```python
from build123d import *

# Parameters (mm, degrees)
P01_CONTACTTOPLEG_START = 37
SK_P01_CONTACTTOPLEG_W  = 25
SK_P01_CONTACTTOPLEG_H  = 24
P01_CONTACTTOPLEG_DEPTH = 3
SK_P02_CONTACTFACE_W    = 3
SK_P02_CONTACTFACE_H    = 24
P02_CONTACTFACE_DEPTH   = 37


with BuildPart() as part:
    # SK_P01_Contacttopleg → P01_Contacttopleg (new body)
    with BuildSketch(Plane(origin=(0, 0, 0), x_dir=(1, 0, 0), z_dir=(0, 1, 0)).offset(P01_CONTACTTOPLEG_START)):
        Rectangle(SK_P01_CONTACTTOPLEG_W, SK_P01_CONTACTTOPLEG_H)
    extrude(amount=P01_CONTACTTOPLEG_DEPTH)

    # SK_P02_Contactface → P02_Contactface (add)
    with BuildSketch(Plane(origin=(0, 0, 0), x_dir=(1, 0, 0), z_dir=(0, 1, 0))):
        with Locations((11, 0)):
            Rectangle(SK_P02_CONTACTFACE_W, SK_P02_CONTACTFACE_H)
    extrude(amount=P02_CONTACTFACE_DEPTH)


solid = part.part
```
Input: part model. Units: mm. Frame: model coordinates. A direction names the side the tool comes from. Round coordinates to 2 decimals unless told otherwise and drop trailing zeros. Order: outer loops, then holes, each group sorted by start corner. A loop starts at its lowest first (then second) coordinate and runs counter-clockwise, first axis right, second up. Notation, with made-up numbers: (-36, 70) - (-10, 70) arc R10 ccw to (-10, 88) - close; hole circle Ø7 at (6.25, 50). An arc over 180 degrees is marked (long way). Answer in a Markdown table with one row per item.
Item 1: Section query B-B (y = 16.5). Return the cut outline in (x, z), then the cut area to 3 significant figures.
Model answer:
| item | result |
|---|---|
| outline | (9.5, -12) - (12.5, -12) - (12.5, 12) - (9.5, 12) - close |
| area | 72.0 mm² |
Item 2: Line query: line 1 (Y direction, x = -2.5, z = 2.75); line 2 (X direction, y = 16, z = 7). Output: solid intervals per line, ascending.
Model answer:
| item | result |
|---|---|
| line 1 | y = 37 to 40 |
| line 2 | x = 9.5 to 12.5 |
Item 3: Pin query (flat end, axial travel): pin 1 (3 mm diameter, centred on x = -9.5, z = 2, fed in from -Y); pin 2 (10 mm diameter, centred on y = 23.5, z = -1, fed in from -X). Return the tip coordinate at first contact, or that it passes through.
Model answer:
| item | result |
|---|---|
| pin 1 | stops at y = 37 |
| pin 2 | stops at x = 9.5 |
Item 4: Section query A-A (z = -8.5). Return the cut outline in (x, y).
Model answer:
| item | result |
|---|---|
| outline | (-12.5, 37) - (9.5, 37) - (9.5, 0) - (12.5, 0) - (12.5, 40) - (-12.5, 40) - close |
Item 5: Section query C-C (x = 1.5). Return the cut outline in (y, z).
Model answer:
| item | result |
|---|---|
| outline | (37, -12) - (40, -12) - (40, 12) - (37, 12) - close |
Item 6: Reachability of faces 1 (the flat face through (-2, 37, 0)), 2 (the flat face through (-12.5, 38, 0)) from +Z, -Z, +X, -X, +Y, -Y: full face, straight path, thin tool, end or side. Return the list, or none.
Model answer:
| item | result |
|---|---|
| face 1 | +Z, -Z, -X, -Y |
| face 2 | +Z, -Z, -X, +Y, -Y |
